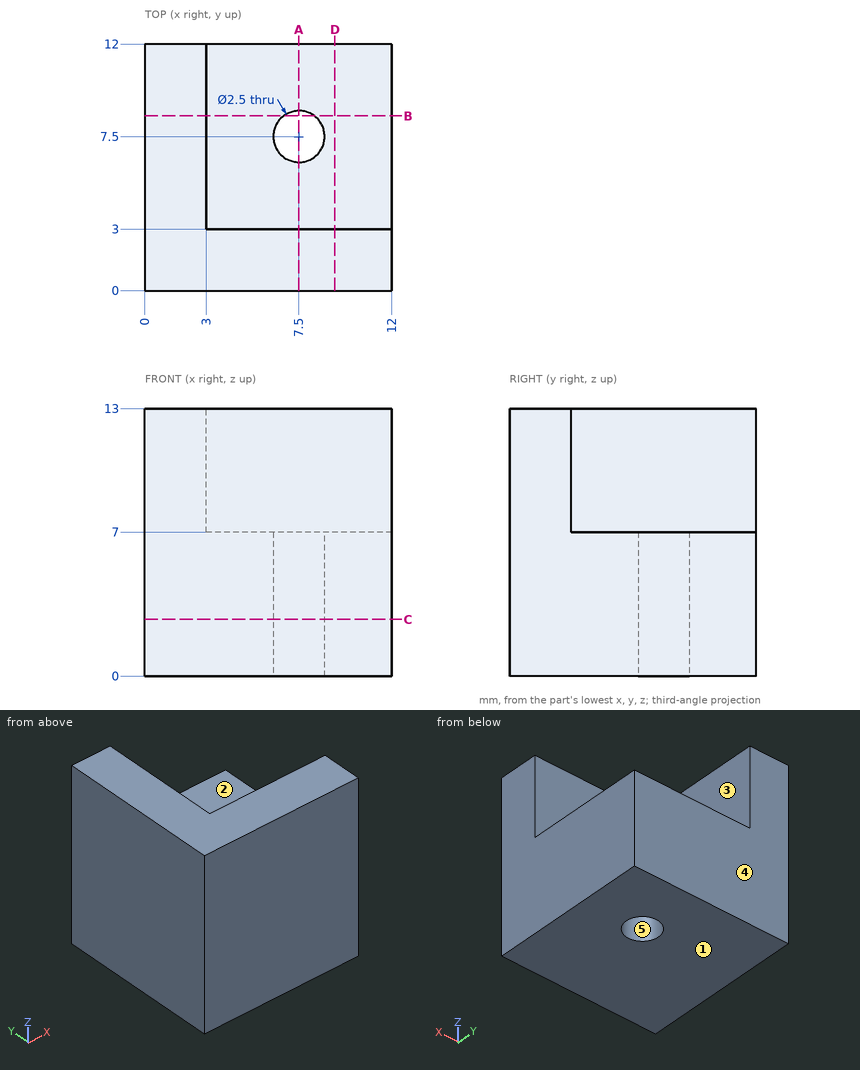
The drawing under review shows one solid part. Ordinate dimensions are in mm from its lowest x, y, z. A direction names the side the tool comes from. Give positions to 0.01 mm unless a question says otherwise; leave off trailing zeros. Write each loop counter-clockwise with the first axis right and the second up, starting at its lowest first coordinate (ties: lowest second). Pieces come first, ordered by that corner, then holes. Notation, with made-up numbers: (68.25, -4.5) -> (72.25, -4.5) arc R25 cw to (72.25, 23.5) -> close; hole circle Ø6 at (84, 62.5). An arc over 180 degrees is marked (long way). Put each result on its own line as item: value.
(1) We need section D-D, the plane x = 9.25. Give the boundary of the cut face in (y, z), and give its area (3 significant figures).
Results are:
outline: (0, 0) -> (12, 0) -> (12, 7) -> (3, 7) -> (3, 13) -> (0, 13) -> close
area: 102 mm²
(2) The part is to be moulded in two halves that separate along Y. For the marked faces 3, 4 and 5, say which applies: pulls with the +Y half, pulls with the -Y half, needs draft (parallel to the pull), parting line crosses it, or undercut.
Results are:
face 3: needs draft
face 4: pulls with the +Y half
face 5: undercut
(3) We need section A-A, the plane x = 7.5. Give the boundary of the cut face in (y, z), and give its area (3 significant figures).
Results are:
outline: (0, 0) -> (6.25, 0) -> (6.25, 7) -> (3, 7) -> (3, 13) -> (0, 13) -> close; (8.75, 0) -> (12, 0) -> (12, 7) -> (8.75, 7) -> close
area: 84.5 mm²
(4) We need section C-C, the plane z = 2.75. Give the boundary of the cut face in (x, y).
Results are:
outline: (0, 0) -> (12, 0) -> (12, 12) -> (0, 12) -> close; hole circle Ø2.5 at (7.5, 7.5)
(5) To check wall thickness, follow probe 1 along Y at (x, z) = (7.5, 1.75); probe 2 along Z at (x, y) = (3.25, 11.5); probe 3 along X at (y, z) = (9.25, 11). State the ranges of each line that lie inside material, in increasing order. Write a range as from..to.
Results are:
probe 1: 0..6.25, 8.75..12
probe 2: 0..7
probe 3: 0..3
(6) For pin 1 Ø5 at (x, z) = (7.5, 10.5) entering from +Y; pin 2 Ø3 at (x, y) = (7.5, 7.5) entering from +Z; pin 3 Ø5 at (y, z) = (6, 10) entering from +X, all flat-tipped, find the tip position at first contact; note any pin that passes through.
Results are:
pin 1: y = 3
pin 2: z = 7
pin 3: x = 3
(7) We need section B-B, the plane y = 8.5. Give the boundary of the cut face in (x, z), and give its area (3 significant figures).
Results are:
outline: (0, 0) -> (6.75, 0) -> (6.75, 7) -> (3, 7) -> (3, 13) -> (0, 13) -> close; (8.25, 0) -> (12, 0) -> (12, 7) -> (8.25, 7) -> close
area: 91.5 mm²
(8) Tool access review of the marked faces 1 and 2: name each direction out of +Z, -Z, +X, -X, +Y, -Y from which nothing blocks a thin tool from reaching the whole face with its end or side.
Results are:
face 1: -Z, +X, -X, +Y, -Y
face 2: +Z, +X, +Y
